from build123d import *

# Parameters (mm, degrees)
SKETCH_1_W                = 90
SKETCH_1_H                = 80
EXTRUDE_1_DEPTH           = 40
SKETCH_10_W               = 60
SKETCH_10_H               = 30
CUT_EXTRUDE_1_DEPTH       = 107.301458127
HOLE_WIZARD_2_D           = 10
CUT_EXTRUDE_2_DEPTH       = 101.124921973
HOLE_WIZARD_1_D           = 5.5
HOLE_WIZARD_1_CBORE_D     = 10
HOLE_WIZARD_1_CBORE_DEPTH = 5.7
HOLE_WIZARD_1_2_D         = 28
HOLE_WIZARD_M6_1_D        = 5


with BuildPart() as part:
    # 草图1 → 凸台-拉伸1 (new body)
    with BuildSketch(Plane(origin=(0, 0, 0), x_dir=(1, 0, 0), z_dir=(0, 1, 0))):
        Rectangle(SKETCH_1_W, SKETCH_1_H)
    extrude(amount=EXTRUDE_1_DEPTH)

    # 草图10 → 切除-拉伸1 (cut, through all)
    with BuildSketch(Plane(origin=(45, 0, 0), x_dir=(0, 0, -1), z_dir=(1, 0, 0))):
        with Locations((0, 15)):
            Rectangle(SKETCH_10_W, SKETCH_10_H)
    extrude(amount=-CUT_EXTRUDE_1_DEPTH, mode=Mode.SUBTRACT)

    # 孔2 (through all)
    with Locations(Plane.XY.offset(40)):
        with Locations((0, 12)):
            Hole(HOLE_WIZARD_2_D / 2)

    # 草图13 → 切除-拉伸2 (cut, through all)
    with BuildSketch(Plane.XY.offset(40)):
        with BuildLine():
            ThreePointArc((-28.343874018, 14.979061203), (-28.5, 12), (-28.343874018, 9.020938797))
            ThreePointArc((-28.343874018, 9.020938797), (-24.497197763, 5.905961785), (-21.38222075, 9.75263804))
            ThreePointArc((-21.38222075, 9.75263804), (-21.5, 12), (-21.38222075, 14.24736196))
            ThreePointArc((-21.38222075, 14.24736196), (-24.497197763, 18.094038215), (-28.343874018, 14.979061203))
        make_face()
        with BuildLine():
            ThreePointArc((21.38222075, 9.75263804), (24.497197763, 5.905961785), (28.343874018, 9.020938797))
            ThreePointArc((28.343874018, 9.020938797), (28.5, 12), (28.343874018, 14.979061203))
            ThreePointArc((28.343874018, 14.979061203), (24.497197763, 18.094038215), (21.38222075, 14.24736196))
            ThreePointArc((21.38222075, 14.24736196), (21.5, 12), (21.38222075, 9.75263804))
        make_face()
    extrude(amount=-CUT_EXTRUDE_2_DEPTH, mode=Mode.SUBTRACT)

    # Hole Wizard 1 (through all)
    with Locations(Plane(origin=(-40.148551056, 30, -46.468490431), x_dir=(-1, 0, 0), z_dir=(0, -1, 0))):
        with Locations((-26.148551056, -60.468490431), (-54.148551056, -60.468490431), (-54.148551056, -32.468490431), (-26.148551056, -32.468490431)):
            CounterBoreHole(HOLE_WIZARD_1_D / 2, HOLE_WIZARD_1_CBORE_D / 2, HOLE_WIZARD_1_CBORE_DEPTH)

    # Hole Wizard 1 2 (through all)
    with Locations(Plane(origin=(0, 0, 0), x_dir=(-1, 0, 0), z_dir=(0, -1, 0))):
        with Locations((0, 0)):
            Hole(HOLE_WIZARD_1_2_D / 2)

    # M6 螺纹孔1 (through all)
    with Locations(Plane(origin=(0, 40, 0), x_dir=(1, 0, 0), z_dir=(0, 1, 0))):
        with Locations((-36, 0), (36, 0)):
            Hole(HOLE_WIZARD_M6_1_D / 2)


solid = part.part
Could you check a few things on this model? Use its own coordinates, in mm. A direction names the side the tool comes from. Give positions to 0.01 mm unless a question says otherwise; leave off trailing zeros. Order: outer loops, then holes, each group sorted by start corner. A loop starts at its lowest first (then second) coordinate and runs counter-clockwise, first axis right, second up. Notation, with made-up numbers: (29, 59.25) -> (55, 59.25) arc R15 cw to (55, 86.25) -> close; hole circle Ø8 at (1, 10.5). An arc over 180 degrees is marked (long way). Answer in a Markdown table with one row per item. Add a question column.
Item 1: Imagine slicing it at C-C (z = 0). List the corners of the cut face in (x, y) for me, and give its area (3 significant figures).
Item 2: Imagine slicing it at A-A (y = 27.5). List the corners of the cut face in (x, z) for me, and give its area (3 significant figures).
Item 3: Please list where these lines run through material, in increasing order: probe 1 along Z at (x, y) = (33, 8.5); probe 2 along Z at (x, y) = (0, 32); probe 3 along Y at (x, z) = (-17, 6.5).
Item 4: Imagine slicing it at D-D (x = 36). List the corners of the cut face in (y, z) for me.
Item 5: We'd pull the mould along Y, two halves only. Please class faces 6 (the flat face through (-1, 20, 40)), 7 (the flat face through (11.8, 35.7, -11.8)), 8 (the cylindrical face through (24.421, 5.915, -34.93)): pulls with the +Y half, pulls with the -Y half, needs draft (parallel to the pull), parting line crosses it, or undercut.
Item 6: I'm going to push flat-ended pins straight in: P1, Ø8, axis at x = 14, z = 13.5, coming from the -Y side; P2, Ø18, axis at x = 20, z = 3.5, coming from the -Y side. Where does each tip first touch, or does it pass through?
Item 7: Imagine slicing it at B-B (y = 12). Count the separate pieces of the cut face and the enclosed holes in it, and give its area (3 significant figures).
Item 8: For faces 1 (the flat face through (45, 33, 1)), 2 (the cylindrical face through (-16.027, 37.88, 12.141)), 3 (the cylindrical face through (11.693, 32.81, -9.564)), 4 (the flat face through (1, 18, 30)), 5 (the cylindrical face through (-28.5, 12, 35.1)), which set-ups out of +Z, -Z, +X, -X, +Y, -Y let a thin tool reach every point of the face, with its end or its side?
Result:
| question | item | result |
|---|---|---|
| 1 | outline | (-45, 30) -> (-38.5, 30) -> (-38.5, 40) -> (-45, 40) -> close; (-33.5, 30) -> (-14, 30) -> (-14, 40) -> (-33.5, 40) -> close; (14, 30) -> (33.5, 30) -> (33.5, 40) -> (14, 40) -> close; (38.5, 30) -> (45, 30) -> (45, 40) -> (38.5, 40) -> close |
| 1 | area | 520 mm2 |
| 2 | outline | (-45, -40) -> (45, -40) -> (45, -30) -> (-45, -30) -> close; (-45, 30) -> (45, 30) -> (45, 40) -> (-45, 40) -> close |
| 2 | area | 1,800 mm2 |
| 3 | probe 1 | -40 to -30, 30 to 40 |
| 3 | probe 2 | -40 to -14, 14 to 40 |
| 3 | probe 3 | 30 to 40 |
| 4 | outline | (0, -40) -> (40, -40) -> (40, -2.5) -> (30, -2.5) -> (30, -30) -> (0, -30) -> close; (0, 30) -> (30, 30) -> (30, 2.5) -> (40, 2.5) -> (40, 40) -> (0, 40) -> close |
| 5 | face 6 | needs draft |
| 5 | face 7 | pulls with the -Y half |
| 5 | face 8 | undercut |
| 6 | P1 | y = 35.7 |
| 6 | P2 | y = 30 |
| 7 | separate pieces | 8 |
| 7 | enclosed holes | 0 |
| 7 | area | 1,320 mm2 |
| 8 | face 1 | +Z, -Z, +X, +Y, -Y |
| 8 | face 2 | +Y, -Y |
| 8 | face 3 | -Y |
| 8 | face 4 | +X, -X, -Y |
| 8 | face 5 | +Z, -Z |
